Design review of the part built by this model. Coordinates are the model's own, in mm. Face numbers are marked on the shaded views. A direction names the side the tool comes from. Coordinates: 2 decimals unless noted, no trailing zeros. Order: outer loops, then holes, each group sorted by start corner. A loop starts at its lowest first (then second) coordinate and runs counter-clockwise, first axis right, second up.
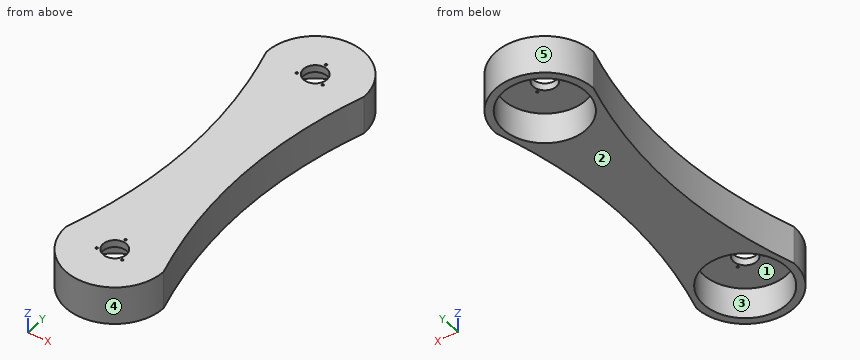
from build123d import *

# Parameters (mm, degrees)
BOSS_EXTRUDE1_DEPTH = 90
SKETCH2_R           = 97.5
CUT_EXTRUDE1_DEPTH  = 72.91
SKETCH4_R           = 2.5
CUT_EXTRUDE3_DEPTH  = 20
SKETCH3_R           = 27.5
CUT_EXTRUDE4_DEPTH  = 20
CIRPATTERN2_COUNT   = 3
SKETCH6_R           = 97.5
CUT_EXTRUDE5_DEPTH  = 72.91
SKETCH7_R           = 27.5
CUT_EXTRUDE6_DEPTH  = 72.91
SKETCH8_R           = 2.5
SKETCH8_R_2         = 27.5
CUT_EXTRUDE7_DEPTH  = 72.91


with BuildPart() as part:
    # Sketch1 → Boss-Extrude1 (new body)
    with BuildSketch(Plane(origin=(0, 0, 0), x_dir=(0, 1, 0), z_dir=(0, 0, 1))):
        with BuildLine():
            ThreePointArc((0, 115), (-115, 0), (0, -115))
            add(Edge.make_bspline(
                [(0, -115), (325, -15), (650, -115)],
                knots=[0, 0, 0, 1, 1, 1], degree=2))
            ThreePointArc((650, -115), (765, 0), (650, 115))
            add(Edge.make_bspline(
                [(0, 115), (325, 15), (650, 115)],
                knots=[0, 0, 0, 1, 1, 1], degree=2))
        make_face()
    extrude(amount=BOSS_EXTRUDE1_DEPTH)

    # Sketch2 → Cut-Extrude1 (cut)
    with BuildSketch(Plane(origin=(0, 0, 0), x_dir=(1, 0, 0), z_dir=(0, 0, -1))):
        with Locations(Location((0, 0, 0), (0, 0, 180))):
            Circle(SKETCH2_R)
    extrude(amount=-CUT_EXTRUDE1_DEPTH, mode=Mode.SUBTRACT)

    # Sketch4 → Cut-Extrude3 (cut)
    with BuildSketch(Plane.XY.offset(90)):
        with Locations((0, 35)):
            Circle(SKETCH4_R)
    cut_extrude3 = extrude(amount=-CUT_EXTRUDE3_DEPTH, mode=Mode.SUBTRACT)

    # Sketch3 → Cut-Extrude4 (cut)
    with BuildSketch(Plane(origin=(0, 0, 72.91), x_dir=(1, 0, 0), z_dir=(0, 0, -1))):
        with Locations(Location((0, 0, 0), (0, 0, 180))):
            Circle(SKETCH3_R)
    extrude(amount=-CUT_EXTRUDE4_DEPTH, mode=Mode.SUBTRACT)

    # CirPattern2: Cut-Extrude3 ×3 about axis
    cirpattern2_axis = Axis((0, 0, 0), (0, 0, 1))
    for i in range(1, CIRPATTERN2_COUNT):
        add(cut_extrude3.rotate(cirpattern2_axis, i * 360 / CIRPATTERN2_COUNT), mode=Mode.SUBTRACT)

    # Sketch6 → Cut-Extrude5 (cut)
    with BuildSketch(Plane(origin=(0, 0, 0), x_dir=(1, 0, 0), z_dir=(0, 0, -1))):
        with Locations(Location((0, -650, 0), (0, 0, 180))):
            Circle(SKETCH6_R)
    extrude(amount=-CUT_EXTRUDE5_DEPTH, mode=Mode.SUBTRACT)

    # Sketch7 → Cut-Extrude6 (cut)
    with BuildSketch(Plane(origin=(0, 0, 72.91), x_dir=(1, 0, 0), z_dir=(0, 0, -1))):
        with Locations(Location((0, -650, 0), (0, 0, 180))):
            Circle(SKETCH7_R)
    extrude(amount=-CUT_EXTRUDE6_DEPTH, mode=Mode.SUBTRACT)

    # Sketch8 → Cut-Extrude7 (cut)
    with BuildSketch(Plane.XY.offset(90)):
        with Locations((-30.310889132, 632.5)):
            Circle(SKETCH8_R)
        with Locations((0, 685)):
            Circle(SKETCH8_R)
        with Locations((30.310889132, 632.5)):
            Circle(SKETCH8_R)
        with Locations(Location((30.310889132, -17.5, 0), (0, 0, 240))):
            Circle(SKETCH8_R)
        with Locations((0, 35)):
            Circle(SKETCH8_R)
        with Locations(Location((-30.310889132, -17.5, 0), (0, 0, 120))):
            Circle(SKETCH8_R)
        with Locations(Location((0, 650, 0), (0, 0, 180))):
            Circle(SKETCH8_R_2)
    extrude(amount=-CUT_EXTRUDE7_DEPTH, mode=Mode.SUBTRACT)


solid = part.part
1. Insertion check: pin 1 (3 mm diameter, centred on x = 30.31, y = 632.5, fed in from +Z); pin 2 (10 mm diameter, centred on y = 155, z = 63.5, fed in from -X); pin 3 (8 mm diameter, centred on x = -30.31, y = 632.5, fed in from +Z); pin 4 (1 mm diameter, centred on x = -23, z = 55, fed in from +Y). Each pin has a flat end and moves straight along its axis. Give the tip position at first contact, or say it passes through.
2. Add section B-B (z = 7.5). State how many separate pieces and enclosed holes the cut face has, and give its area (3 significant figures).
3. Add section A-A (x = -49). Give the boundary of the cut face in (y, z), and give its area (3 significant figures).
4. To check wall thickness, follow line 1 (Y direction, x = 0, z = 82.75); line 2 (Y direction, x = -18, z = 29); line 3 (X direction, y = -17, z = 83). State the ranges of each line that lie inside material, in increasing order.
5. For the marked faces 1 and 2, list the 3-axis set-ups (+Z, -Z, +X, -X, +Y, -Y) from which the entire face can be reached by the end or side of a thin tool; tool diameter is ignored.
6. Mouldability with a two-part tool opening along Y and no side actions: class the marked faces 3, 4 and 5 as pulls with the +Y half, pulls with the -Y half, needs draft (parallel to the pull), parting line crosses it, or undercut.
Solution:
1. pin 1: passes through
1. pin 2: stops at x = -79.5
1. pin 3: stops at z = 90
1. pin 4: stops at y = 762.78
2. separate pieces: 1
2. enclosed holes: 2
2. area: 88,000 mm2
3. outline: (-104.04, 0) - (-84.29, 0) - (-84.29, 72.91) - (84.29, 72.91) - (84.29, 0) - (565.71, 0) - (565.71, 72.91) - (734.29, 72.91) - (734.29, 0) - (754.04, 0) - (754.04, 90) - (-104.04, 90) - close
3. area: 52,600 mm2
4. line 1: y = -115 to -27.5, 27.5 to 32.5, 37.5 to 622.5, 677.5 to 682.5, 687.5 to 765
4. line 2: y = -113.58 to -95.82, 95.82 to 554.18, 745.82 to 763.58
4. line 3: x = -113.74 to -32.76, -27.86 to -21.62, 21.62 to 27.86, 32.76 to 113.74
5. face 1: -Z
5. face 2: -Z, +X, -X, +Y, -Y
6. face 3: undercut
6. face 4: pulls with the -Y half
6. face 5: pulls with the +Y half
